Can you work these out from the model? Positions are in its coordinate system, mm. Face numbers are marked on the shaded views. A direction names the side the tool comes from. Give positions to 0.01 mm unless a question says otherwise; leave off trailing zeros. Order: outer loops, then holes, each group sorted by start corner. A loop starts at its lowest first (then second) coordinate and runs counter-clockwise, first axis right, second up. Notation, with made-up numbers: (-21, 79.5) - (29, 79.5) arc R6 cw to (29, 88.5) - close; hole circle Ø3 at (-14.5, 29). An arc over 180 degrees is marked (long way). One line per question, with ' | ' between items.
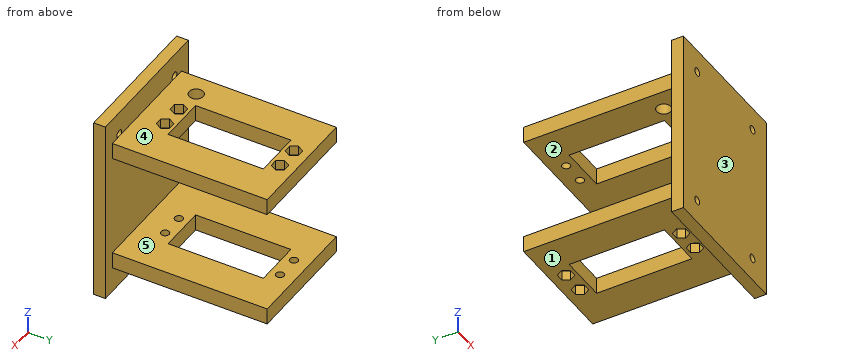
```python
from build123d import *

# Parameters (mm, degrees)
SKETCH1_W           = 60
SKETCH1_H           = 80
BOSS_EXTRUDE1_DEPTH = 2.5
SKETCH2_R           = 1.725
CUT_EXTRUDE1_DEPTH  = 51.249378106
SKETCH3_W           = 50
SKETCH3_H           = 66
BOSS_EXTRUDE2_DEPTH = 7
SKETCH4_W           = 19.9
SKETCH4_H           = 40.6
CUT_EXTRUDE2_DEPTH  = 102.750921372
SKETCH5_R           = 1.725
CUT_EXTRUDE3_DEPTH  = 102.750921372
CUT_EXTRUDE4_DEPTH  = 4.2
CUT_EXTRUDE5_START  = 21
SKETCH7_R           = 3
CUT_EXTRUDE5_DEPTH  = 9


with BuildPart() as part:
    # Sketch1 → Boss-Extrude1 (new, symmetric)
    with BuildSketch(Plane(origin=(0, 0, 0), x_dir=(1, 0, 0), z_dir=(0, 1, 0))):
        Rectangle(SKETCH1_W, SKETCH1_H)
    extrude(amount=BOSS_EXTRUDE1_DEPTH, both=True)

    # Sketch2 → Cut-Extrude1 (cut, through all)
    with BuildSketch(Plane(origin=(0, 2.5, 0), x_dir=(1, 0, 0), z_dir=(0, 1, 0))):
        with Locations(Location((-20, 30, 0), (0, 0, 270))):
            Circle(SKETCH2_R)
        with Locations(Location((20, 30, 0), (0, 0, 270))):
            Circle(SKETCH2_R)
        with Locations(Location((20, -30, 0), (0, 0, 270))):
            Circle(SKETCH2_R)
        with Locations(Location((-20, -30, 0), (0, 0, 270))):
            Circle(SKETCH2_R)
    extrude(amount=-CUT_EXTRUDE1_DEPTH, mode=Mode.SUBTRACT)

    # Sketch3 → Boss-Extrude2 (add)
    with BuildSketch(Plane.XY.offset(22)):
        with Locations((0, 35.5)):
            Rectangle(SKETCH3_W, SKETCH3_H)
    boss_extrude2 = extrude(amount=BOSS_EXTRUDE2_DEPTH)

    # Mirror1: Boss-Extrude2 across plane
    add(boss_extrude2.mirror(Plane.XY))

    # Sketch4 → Cut-Extrude2 (cut, through all)
    with BuildSketch(Plane.XY.offset(29)):
        with Locations((0, 37.7)):
            Rectangle(SKETCH4_W, SKETCH4_H)
    extrude(amount=-CUT_EXTRUDE2_DEPTH, mode=Mode.SUBTRACT)

    # Sketch5 → Cut-Extrude3 (cut, through all)
    with BuildSketch(Plane.XY.offset(29)):
        with Locations((-5, 62.2)):
            Circle(SKETCH5_R)
        with Locations((5, 62.2)):
            Circle(SKETCH5_R)
        with Locations((-5, 13.2)):
            Circle(SKETCH5_R)
        with Locations((5, 13.2)):
            Circle(SKETCH5_R)
    extrude(amount=-CUT_EXTRUDE3_DEPTH, mode=Mode.SUBTRACT)

    # Sketch6 → Cut-Extrude4 (cut)
    with BuildSketch(Plane.XY.offset(29)):
        Polygon((-1.766838493, 62.2), (-3.383419246, 65), (-6.616580754, 65), (-8.233161507, 62.2), (-6.616580754, 59.4), (-3.383419246, 59.4), align=None)
        Polygon((1.766838493, 62.2), (3.383419246, 59.4), (6.616580754, 59.4), (8.233161507, 62.2), (6.616580754, 65), (3.383419246, 65), align=None)
        Polygon((-1.766838493, 13.2), (-3.383419246, 16), (-6.616580754, 16), (-8.233161507, 13.2), (-6.616580754, 10.4), (-3.383419246, 10.4), align=None)
        Polygon((8.233161507, 13.2), (6.616580754, 16), (3.383419246, 16), (1.766838493, 13.2), (3.383419246, 10.4), (6.616580754, 10.4), align=None)
    cut_extrude4 = extrude(amount=-CUT_EXTRUDE4_DEPTH, mode=Mode.SUBTRACT)

    # Mirror3: Cut-Extrude4 across plane
    add(cut_extrude4.mirror(Plane.XY), mode=Mode.SUBTRACT)

    # Sketch7 → Cut-Extrude5 (cut)
    with BuildSketch(Plane.XY.offset(CUT_EXTRUDE5_START)):
        with Locations(Location((-16, 14.1, 0), (0, 0, 180))):
            Circle(SKETCH7_R)
    extrude(amount=CUT_EXTRUDE5_DEPTH, mode=Mode.SUBTRACT)


solid = part.part
```
(1) Imagine slicing it at C-C (x = -20). List the corners of the cut face in (y, z) for me (3 decimals).
Answer below:
outline: (-2.5, -40) - (2.5, -40) - (2.5, -31.725) - (-2.5, -31.725) - close; (-2.5, -28.275) - (2.5, -28.275) - (2.5, -29) - (68.5, -29) - (68.5, -22) - (2.5, -22) - (2.5, 22) - (68.5, 22) - (68.5, 29) - (2.5, 29) - (2.5, 28.275) - (-2.5, 28.275) - close; (-2.5, 31.725) - (2.5, 31.725) - (2.5, 40) - (-2.5, 40) - close
(2) Will these pins go through, and if not, where does the flat tip stop? pin 1 (5 mm diameter, centred on x = -7.5, y = 55.5, fed in from -Z); pin 2 (4.5 mm diameter, centred on x = 3.5, y = 12, fed in from +Z); pin 3 (10 mm diameter, centred on x = -3.5, y = 41, fed in from -Z); pin 4 (3 mm diameter, centred on x = -6, y = 14, fed in from +Z).
Answer below:
pin 1: z = -29 | pin 2: z = 29 | pin 3: through | pin 4: z = 24.8
(3) Imagine slicing it at B-B (y = 35). List the corners of the cut face in (x, z) for me.
Answer below:
outline: (-25, -29) - (-9.95, -29) - (-9.95, -22) - (-25, -22) - close; (-25, 22) - (-9.95, 22) - (-9.95, 29) - (-25, 29) - close; (9.95, -29) - (25, -29) - (25, -22) - (9.95, -22) - close; (9.95, 22) - (25, 22) - (25, 29) - (9.95, 29) - close
(4) On a 3-axis mill with a long thin cutter (end or side, diameter ignored), from which of +Z, -Z, +X, -X, +Y, -Y can I reach the whole of each face in a straight line? I mean the marked faces 4 and 5. Say none if no direction works.
Answer below:
face 4: +Z, +X, -X, +Y | face 5: +X, -X, +Y
(5) Imagine slicing it at A-A (z = -30). List the corners of the cut face in (x, y) for me (3 decimals), and give its area (4 significant figures).
Answer below:
outline: (-30, -2.5) - (-21.725, -2.5) - (-21.725, 2.5) - (-30, 2.5) - close; (-18.275, -2.5) - (18.275, -2.5) - (18.275, 2.5) - (-18.275, 2.5) - close; (21.725, -2.5) - (30, -2.5) - (30, 2.5) - (21.725, 2.5) - close | area: 265.5 mm^2
(6) If I drill on line 1 (Y direction, x = 5, z = 23) (3 decimals); line 2 (Z direction, x = 20, y = 1.05) (3 decimals); line 3 (Y direction, x = -9, z = -27), over which ranges is the centre line in solid material (lowest first)?
Answer below:
line 1: -2.5 to 11.475, 14.925 to 17.4, 58 to 60.475, 63.925 to 68.5 | line 2: -40 to -31.725, -28.275 to 28.275, 31.725 to 40 | line 3: -2.5 to 17.4, 58 to 68.5
(7) If we mould it in two halves opening along Z, with no side actions, what happens to the marked faces 1, 2 and 3? For each: released by +Z, released by -Z, zero draft, split by the parting line, or undercut.
Answer below:
face 1: released by -Z | face 2: undercut | face 3: zero draft
(8) Imagine slicing it at D-D (x = -11). List the corners of the cut face in (y, z) for me.
Answer below:
outline: (-2.5, -40) - (2.5, -40) - (2.5, -29) - (68.5, -29) - (68.5, -22) - (2.5, -22) - (2.5, 22) - (68.5, 22) - (68.5, 29) - (2.5, 29) - (2.5, 40) - (-2.5, 40) - close
